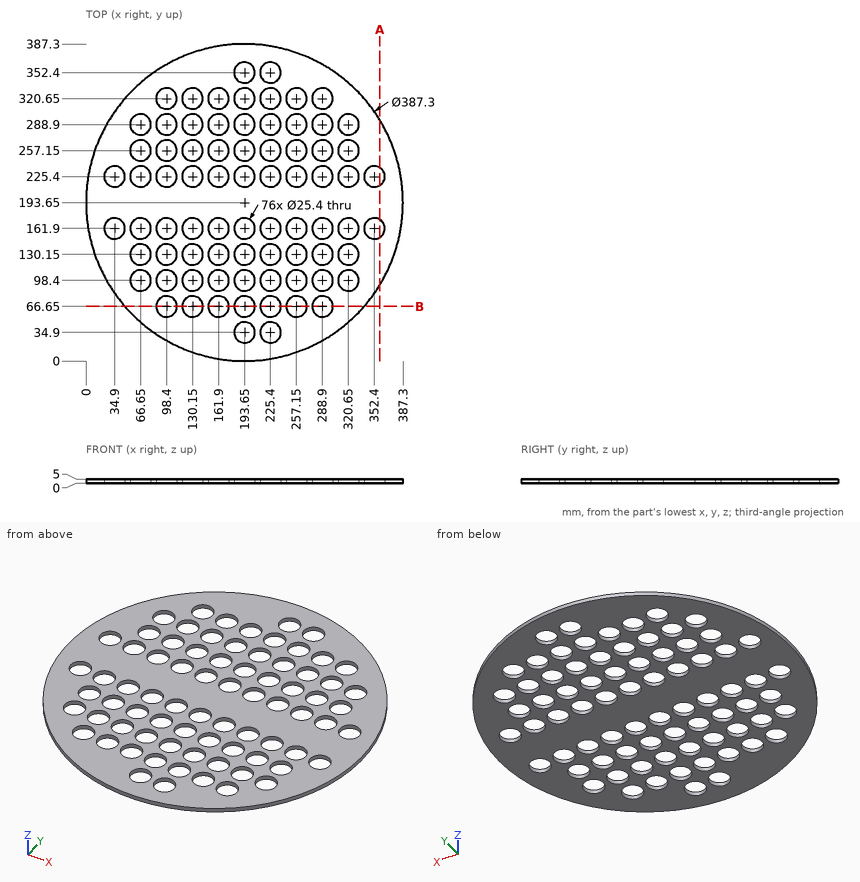
Geometry check sheet. Reference: drawing and pictorial views, mm from the part's lowest x, y, z. Coordinates: 2 decimals unless noted, no trailing zeros. Order: outer loops, then holes, each group sorted by start corner. A loop starts at its lowest first (then second) coordinate and runs counter-clockwise, first axis right, second up. Notation, with made-up numbers: M -28,48.25 L 8,48.25 A26 cw 8,71.25 Z; hole C -29,-20.5 d5. An arc over 180 degrees is marked long. Write each question's results on one line, items separated by ' | '. Start each with the question number.
1. Cross-section at B-B on y = 66.65. State how many separate pieces and enclosed holes the cut face has, and give its area (3 significant figures).
2. Material ranges on probe 1 along Y at (x, z) = (32, 0.8); probe 2 along Y at (x, z) = (302.5, 1.8); probe 3 along X at (y, z) = (83.5, 4.65), recorded low to high.
3. Cross-section at A-A on x = 359. Record the cut outline in (y, z).
4. Go/stop test with flat-tipped pins: P1, Ø23, axis at x = 225.4, y = 130.15, coming from the -Z side; P2, Ø3, axis at x = 40.5, z = 2, coming from the -Y side. Record where each tip stops, or that it passes through.
Checks:
1) separate pieces: 8 | enclosed holes: 0 | area: 573 mm²
2) probe 1: y = 87.02 to 149.54, 174.26 to 213.04, 237.76 to 300.28 | probe 2: y = 33.49 to 353.81 | probe 3: x = 34.38 to 352.92
3) outline: M 92.85,0 L 151.05,0 L 151.05,5 L 92.85,5 Z; M 172.75,0 L 214.55,0 L 214.55,5 L 172.75,5 Z; M 236.25,0 L 294.45,0 L 294.45,5 L 236.25,5 Z
4) P1: passes through | P2: stops at y = 73.22
